Could you check a few things on this model? Use its own coordinates, in mm. Face numbers are marked on the shaded views. A direction names the side the tool comes from. Coordinates: 2 decimals unless noted, no trailing zeros. Loops run counter-clockwise (first coordinate to the right, second up) from the corner with the lowest first, then second, coordinate; pieces in that order, holes last.
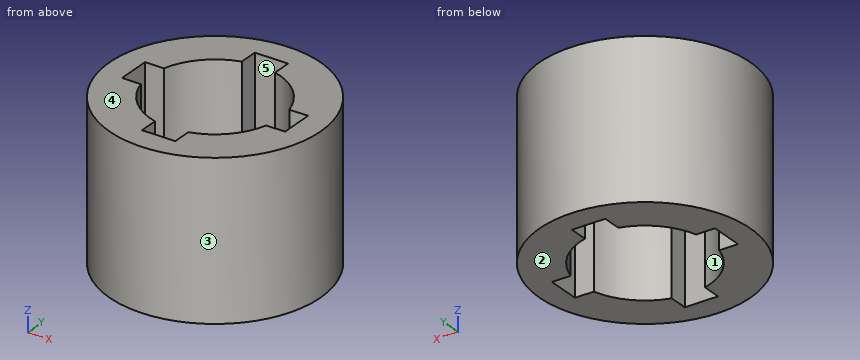
from build123d import *

# Parameters (mm, degrees)
SKETCH1_R           = 9.5
BOSS_EXTRUDE1_DEPTH = 14


with BuildPart() as part:
    # Sketch1 → Boss-Extrude1 (new body)
    with BuildSketch(Plane.XY):
        Circle(SKETCH1_R)
        with BuildLine():
            Line((-1.5, 5.652839314), (-1.5, 7.348469228))
            Line((-1.5, 7.348469228), (1.5, 7.348469228))
            Line((1.5, 7.348469228), (1.5, 5.652839314))
            ThreePointArc((1.5, 5.652839314), (4.135492251, 4.135492251), (5.652839314, 1.5))
            Line((5.652839314, 1.5), (7.348469228, 1.5))
            Line((7.348469228, 1.5), (7.348469228, -1.5))
            Line((7.348469228, -1.5), (5.652839314, -1.5))
            ThreePointArc((5.652839314, -1.5), (4.135492251, -4.135492251), (1.5, -5.652839314))
            Line((1.5, -5.652839314), (1.5, -7.348469228))
            Line((1.5, -7.348469228), (-1.5, -7.348469228))
            Line((-1.5, -7.348469228), (-1.5, -5.652839314))
            ThreePointArc((-1.5, -5.652839314), (-4.135492251, -4.135492251), (-5.652839314, -1.5))
            Line((-5.652839314, -1.5), (-7.348469228, -1.5))
            Line((-7.348469228, -1.5), (-7.348469228, 1.5))
            Line((-7.348469228, 1.5), (-5.652839314, 1.5))
            ThreePointArc((-5.652839314, 1.5), (-4.135492251, 4.135492251), (-1.5, 5.652839314))
        make_face(mode=Mode.SUBTRACT)
    extrude(amount=BOSS_EXTRUDE1_DEPTH)


solid = part.part
(1) Which directions (+Z, -Z, +X, -X, +Y, -Y) give clear straight access to the entire face, cutting with the end or side of a thin tool? Please do the marked faces 4 and 5.
Answers:
face 4: +Z, +X, -X, +Y, -Y
face 5: +Z, -Z
(2) I need wall thicknesses on probe 1 along Y at (x, z) = (0.25, 3.5); probe 2 along Y at (x, z) = (-4.75, 5.75); probe 3 along X at (y, z) = (1, 7.5). Which ranges of each line are inside material? Lowest first, please.
Answers:
probe 1: y = -9.5 to -7.35, 7.35 to 9.5
probe 2: y = -8.23 to -3.41, 3.41 to 8.23
probe 3: x = -9.45 to -7.35, 7.35 to 9.45
(3) Imagine slicing it at C-C, the plane z = 4.5. Write out the boundary of the cut face in (x, y), and give its area (3 significant figures).
Answers:
outline: circle Ø19 at (0, 0); hole (-7.35, -1.5) - (-5.65, -1.5) arc R5.85 ccw to (-1.5, -5.65) - (-1.5, -7.35) - (1.5, -7.35) - (1.5, -5.65) arc R5.85 ccw to (5.65, -1.5) - (7.35, -1.5) - (7.35, 1.5) - (5.65, 1.5) arc R5.85 ccw to (1.5, 5.65) - (1.5, 7.35) - (-1.5, 7.35) - (-1.5, 5.65) arc R5.85 ccw to (-5.65, 1.5) - (-7.35, 1.5) - close
area: 157 mm2
(4) We'd pull the mould along X, two halves only. Please class the marked faces 1, 2 and 3: +X half, -X half, draft (parallel to the pull), parting line (faces both ways), or undercut.
Answers:
face 1: undercut
face 2: draft
face 3: parting line
(5) For pin 1 (2 mm diameter, centred on x = 7, z = 12, fed in from -Y); pin 2 (0.5 mm diameter, centred on y = -6, z = 7, fed in from -X); pin 3 (1.9 mm diameter, centred on x = 7, z = 9, fed in from -Y), each with a flat end and sliding along its axis, tell me the tip position at first contact or that it passes through.
Answers:
pin 1: stops at y = -7.37
pin 2: stops at x = -7.56
pin 3: stops at y = -7.32
(6) Imagine slicing it at D-D, the plane x = 8.25. Write out the boundary of the cut face in (y, z), and give its area (3 significant figures).
Answers:
outline: (-4.71, 0) - (4.71, 0) - (4.71, 14) - (-4.71, 14) - close
area: 132 mm2
(7) Imagine slicing it at A-A, the plane y = 0. Write out the boundary of the cut face in (x, z), and give its area (3 significant figures).
Answers:
outline: (-9.5, 0) - (-7.35, 0) - (-7.35, 14) - (-9.5, 14) - close; (7.35, 0) - (9.5, 0) - (9.5, 14) - (7.35, 14) - close
area: 60.2 mm2
